The model under review builds one solid part; all positions refer to its coordinate system, in mm. A direction names the side the tool comes from. Round coordinates to 2 decimals unless told otherwise and drop trailing zeros. Loops run counter-clockwise (first coordinate to the right, second up) from the corner with the lowest first, then second, coordinate; pieces in that order, holes last. Notation, with made-up numbers: M -40,-24.5 L 0,-24.5 A15 ccw 0,-9.5 Z; hole C -23.75,0.25 d6. An arc over 180 degrees is marked long. One line per question, with ' | ' between items.
from build123d import *

# Parameters (mm, degrees)
SKETCH1_R           = 1.6
BOSS_EXTRUDE1_DEPTH = 2
SKETCH3_W           = 29.5
SKETCH3_H           = 15
SKETCH3_R           = 2
BOSS_EXTRUDE2_DEPTH = 11.638171
BOSS_EXTRUDE3_REACH = 45.79
SKETCH1_2_R         = 1.6
SKETCH3_2_W         = 29.5
SKETCH3_2_H         = 15
SKETCH3_2_R         = 2
BOSS_EXTRUDE4_DEPTH = 12.458742
CUT_EXTRUDE1_DEPTH  = 4


with BuildPart() as part:
    # Sketch1 → Boss-Extrude1 (new body)
    with BuildSketch(Plane.XY):
        with BuildLine():
            Line((-32.88, 10.023123532), (-29.5, 10.023123532))
            Line((-29.5, 10.023123532), (-29.5, 13))
            Line((-29.5, 13), (0, 13))
            Line((0, 13), (0, 10.023123532))
            Line((0, 10.023123532), (3.38, 10.023123532))
            ThreePointArc((3.38, 10.023123532), (7.518209124, 6.273123532), (3.38, 2.523123532))
            Line((3.38, 2.523123532), (0, 2.523123532))
            Line((0, 2.523123532), (0, 1.167746206))
            Line((0, 1.167746206), (-29.5, 1.167746206))
            Line((-29.5, 1.167746206), (-29.5, 2.523123532))
            Line((-29.5, 2.523123532), (-32.88, 2.523123532))
            ThreePointArc((-32.88, 2.523123532), (-37.018209124, 6.273123532), (-32.88, 10.023123532))
        make_face()
        with Locations((-33.25, 6.273123532)):
            Circle(SKETCH1_R, mode=Mode.SUBTRACT)
        with Locations((3.75, 6.273123532)):
            Circle(SKETCH1_R, mode=Mode.SUBTRACT)
    extrude(amount=BOSS_EXTRUDE1_DEPTH)


with BuildPart() as body_2:
    # Sketch3 → Boss-Extrude2 (new body)
    with BuildSketch(Plane(origin=(0, 1.387555227, 0.371794302), x_dir=(1, 0, 0), z_dir=(0, 0.9659258262890684, 0.2588190451025204))):
        with Locations((-14.75, -9.129616695)):
            Rectangle(SKETCH3_W, SKETCH3_H)
        with Locations(Location((-4.75, -9.129616695, 0), (0, 0, 270))):
            Circle(SKETCH3_R, mode=Mode.SUBTRACT)
        with Locations(Location((-24.75, -9.129616695, 0), (0, 0, 270))):
            Circle(SKETCH3_R, mode=Mode.SUBTRACT)
    extrude(amount=BOSS_EXTRUDE2_DEPTH)

    # Boss-Extrude3: up to this face of the body (flat: up to its plane)
    boss_extrude3_end = Plane(body_2.part.faces().sort_by_distance((-14.75, 6.58658436, 3.451973307))[0])
    # Sketch1<2> → Boss-Extrude3 (add, up to the picked face)
    with BuildSketch(Plane.XY, mode=Mode.PRIVATE) as boss_extrude3_sk1:
        with BuildLine():
            Line((-32.88, 10.023123532), (-29.5, 10.023123532))
            Line((-29.5, 10.023123532), (-29.5, 13))
            Line((-29.5, 13), (0, 13))
            Line((0, 13), (0, 10.023123532))
            Line((0, 10.023123532), (3.38, 10.023123532))
            ThreePointArc((3.38, 10.023123532), (7.518209124, 6.273123532), (3.38, 2.523123532))
            Line((3.38, 2.523123532), (0, 2.523123532))
            Line((0, 2.523123532), (0, 1.167746206))
            Line((0, 1.167746206), (-29.5, 1.167746206))
            Line((-29.5, 1.167746206), (-29.5, 2.523123532))
            Line((-29.5, 2.523123532), (-32.88, 2.523123532))
            ThreePointArc((-32.88, 2.523123532), (-37.018209124, 6.273123532), (-32.88, 10.023123532))
        make_face()
        with Locations(Location((-33.25, 6.273123532, 0), (0, 0, 270))):
            Circle(SKETCH1_2_R, mode=Mode.SUBTRACT)
        with Locations(Location((3.75, 6.273123532, 0), (0, 0, 270))):
            Circle(SKETCH1_2_R, mode=Mode.SUBTRACT)
    boss_extrude3_tool1 = split(extrude(boss_extrude3_sk1.sketch, amount=BOSS_EXTRUDE3_REACH, mode=Mode.PRIVATE), bisect_by=boss_extrude3_end, keep=Keep.BOTH, mode=Mode.PRIVATE)

    add(part.part)  # Boss-Extrude3 merges part
    add(boss_extrude3_tool1.solids().sort_by(Axis((-14.75, 6.925418, 0), (0, 0, 1)))[0])

    # Sketch3<2> → Boss-Extrude4 (add)
    with BuildSketch(Plane(origin=(0, 1.387555227, 0.371794302), x_dir=(1, 0, 0), z_dir=(0, 0.9659258262890684, 0.2588190451025204))):
        with Locations((-14.75, -9.129616695)):
            Rectangle(SKETCH3_2_W, SKETCH3_2_H)
        with Locations(Location((-4.75, -9.129616695, 0), (0, 0, 270))):
            Circle(SKETCH3_2_R, mode=Mode.SUBTRACT)
        with Locations(Location((-24.75, -9.129616695, 0), (0, 0, 270))):
            Circle(SKETCH3_2_R, mode=Mode.SUBTRACT)
    extrude(amount=BOSS_EXTRUDE4_DEPTH)

    # Sketch4 → Cut-Extrude1 (cut)
    with BuildSketch(Plane(origin=(0, 13.421775837, 3.596353996), x_dir=(1, 0, 0), z_dir=(0, 0.9659258262890684, 0.2588190451025205))):
        Polygon((-1.35, -11.09260761), (-1.35, -7.166625779), (-4.75, -5.203634864), (-8.15, -7.166625779), (-8.15, -11.09260761), (-4.75, -13.055598525), align=None)
        Polygon((-21.35, -7.166625779), (-24.75, -5.203634864), (-28.15, -7.166625779), (-28.15, -11.09260761), (-24.75, -13.055598525), (-21.35, -11.09260761), align=None)
    extrude(amount=-CUT_EXTRUDE1_DEPTH, mode=Mode.SUBTRACT)


solid = body_2.part
1) Machinability: for faces 1 (the flat face through (-6.47, 8.4, 14.74)), 2 (the flat face through (-28.15, 9, 12)), 3 (the flat face through (-14, 7, 0)), which of the approach directions +Z, -Z, +X, -X, +Y, -Y give a long, thin tool a straight path to every point of the face, cutting with its end or side? Answer none if there is none.
Output values:
face 1: +Y | face 2: none | face 3: -Z, +X, -X, +Y, -Y
2) Add section B-B on y = 7.25. State how many separate pieces and enclosed holes the cut face has, then the cut area to 3 significant figures.
Output values:
separate pieces: 3 | enclosed holes: 2 | area: 545 mm²
3) Insertion check: P1, Ø5, axis at x = -24.5, z = 12, coming from the -Y side; P2, Ø8, axis at y = 2, z = 8.5, coming from the +X side; P3, Ø1, axis at x = -15, z = 1, coming from the -Y side. Each pin has a flat end and moves straight along its axis. Give the tip position at first contact, or say it passes through.
Output values:
P1: stops at y = -2.4 | P2: stops at x = 0 | P3: stops at y = 1.17
4) Add section D-D on x = -27.5. State the section outline as (y, z) points, then the cut area to 3 significant figures.
Output values:
outline: M -2.92,16.43 L 0.97,1.95 L 1.17,2 L 1.17,0 L 13,0 L 13,5.17 L 11.66,10.16 L 7.8,9.12 L 6.59,13.64 L 10.45,14.67 L 9.12,19.66 Z | area: 211 mm²
5) Add section C-C on z = 17.75. State the section outline as (x, y) points.
Output values:
outline: M -29.5,1.99 L 0,1.99 L 0,9.63 L -29.5,9.63 Z
6) Mouldability with a two-part tool opening along Z and no side actions: class faces 4 (the flat face through (-1.35, 9, 12)), 5 (the flat face through (-14.956, 11.086, 12.313)), 6 (the flat face through (-31, 2.523, 1)) as +Z half, -Z half, draft (parallel to the pull), parting line (faces both ways), or undercut.
Output values:
face 4: undercut | face 5: +Z half | face 6: draft
7) For line 1 (X direction, y = 10.5, z = 11.75); line 2 (Y direction, x = 3.75, z = 1.15); line 3 (X direction, y = 8.25, z = 9.25), list the stretches that pass through material, from the lowest coordinate up.
Output values:
line 1: x = -29.5 to -28.15, -21.35 to -8.15, -1.35 to 0 | line 2: y = 2.5 to 4.67, 7.87 to 10.04 | line 3: x = -29.5 to -27.51, -21.99 to -7.51, -1.99 to 0
8) Add section A-A on x = -10.5. State the section outline as (y, z) points, then the cut area to 3 significant figures.
Output values:
outline: M -2.92,16.43 L 0.97,1.95 L 1.17,2 L 1.17,0 L 13,0 L 13,5.17 L 9.12,19.66 Z | area: 229 mm²
